from build123d import *

# Parameters (mm, degrees)
SKETCH1_R               = 6
BOSS_EXTRUDE1_DEPTH     = 60
SKETCH1_3_R             = 10
BOSS_EXTRUDE2_DEPTH     = 5
CUT_EXTRUDE1_DEPTH      = 62.64414003
CUT_EXTRUDE1_DEPTH_BACK = 62.64414003
SKETCH2_R               = 1.25


with BuildPart() as part:
    # Sketch1 → Boss-Extrude1 (new body)
    with BuildSketch(Plane(origin=(0, 0, 0), x_dir=(1, 0, 0), z_dir=(0, 1, 0))):
        with Locations(Location((0, 0, 0), (0, 0, 270))):
            Circle(SKETCH1_R)
    extrude(amount=BOSS_EXTRUDE1_DEPTH)

    # Sketch1_3 → Boss-Extrude2 (add)
    with BuildSketch(Plane(origin=(0, 0, 0), x_dir=(1, 0, 0), z_dir=(0, 1, 0))):
        with Locations(Location((0, 0, 0), (0, 0, 270))):
            Circle(SKETCH1_3_R)
    extrude(amount=-BOSS_EXTRUDE2_DEPTH)

    # Sketch2 → Cut-Extrude1 (cut, two sides: drawn at the far end of the back side and taken through both)
    with BuildSketch(Plane(origin=(0, 0, 0), x_dir=(0, 0, -1), z_dir=(1, 0, 0)).offset(-CUT_EXTRUDE1_DEPTH_BACK)):
        with Locations((0, 57.5)):
            Circle(SKETCH2_R)
    extrude(amount=CUT_EXTRUDE1_DEPTH + CUT_EXTRUDE1_DEPTH_BACK, mode=Mode.SUBTRACT)


solid = part.part
Verification items for the finished model (mm, model axes). A direction names the side the tool comes from. Give positions to 0.01 mm unless a question says otherwise; leave off trailing zeros. Loops run counter-clockwise (first coordinate to the right, second up) from the corner with the lowest first, then second, coordinate; pieces in that order, holes last.
1. Cross-section at B-B on y = 57.5. Record the cut outline in (x, z), and give its area (3 significant figures).
Derived:
outline: (-5.87, -1.25) arc R6 ccw to (5.87, -1.25) - close; (-5.87, 1.25) - (5.87, 1.25) arc R6 ccw to start
area: 83.3 mm2
2. Cross-section at C-C on z = -3.5. Record the cut outline in (x, y), and give its area (3 significant figures).
Derived:
outline: (-9.37, -5) - (9.37, -5) - (9.37, 0) - (4.87, 0) - (4.87, 60) - (-4.87, 60) - (-4.87, 0) - (-9.37, 0) - close
area: 678 mm2
3. Material ranges on probe 1 along Y at (x, z) = (-0.25, 0); probe 2 along Z at (x, y) = (1.25, 57.5); probe 3 along Z at (x, y) = (-3.25, 57.5), recorded low to high.
Derived:
probe 1: y = -5 to 56.25, 58.75 to 60
probe 2: z = -5.87 to -1.25, 1.25 to 5.87
probe 3: z = -5.04 to -1.25, 1.25 to 5.04
4. Cross-section at D-D on x = 0. Record the cut outline in (y, z).
Derived:
outline: (-5, -10) - (0, -10) - (0, -6) - (60, -6) - (60, 6) - (0, 6) - (0, 10) - (-5, 10) - close; hole circle Ø2.5 at (57.5, 0)
5. Tool access check on faces 4 (the flat face through (-7, 0, 0)), 5 (the flat face through (0, -5, 0)). Record the directions out of +Z, -Z, +X, -X, +Y, -Y that give a thin tool (end or side, any length) a straight path to the whole face; none if there is none.
Derived:
face 4: +Y
face 5: +Z, -Z, +X, -X, -Y
6. Go/stop test with flat-tipped pins: P1, Ø1, axis at x = 1, y = 5, coming from the -Z side; P2, Ø2, axis at y = 52, z = -5.5, coming from the -X side; P3, Ø3, axis at x = -3.5, y = 27, coming from the +Z side. Record where each tip stops, or that it passes through.
Derived:
P1: stops at z = -5.98
P2: stops at x = -3.97
P3: stops at z = 5.66
7. Release check for a two-part mould opening along Z. For faces 1 (the cylindrical face through (1.802, 29.58, 5.723)), 2 (the cylindrical face through (-0.08, 58.74, 0.16)), 3 (the flat face through (0, 60, 0)) record: +Z half, -Z half, draft (parallel to the pull), parting line (faces both ways), or undercut.
Derived:
face 1: parting line
face 2: undercut
face 3: draft
8. Cross-section at A-A on x = -3.5. Record the cut outline in (y, z).
Derived:
outline: (-5, -9.37) - (0, -9.37) - (0, -4.87) - (60, -4.87) - (60, 4.87) - (0, 4.87) - (0, 9.37) - (-5, 9.37) - close; hole circle Ø2.5 at (57.5, 0)
